from build123d import *

# Parameters (mm, degrees)
SKETCH_1_W                  = 56
SKETCH_1_H                  = 54
SKETCH_1_R                  = 5
EXTRUDE_1_DEPTH             = 9.2
HOLE_WIZARD_M2_1_AT_2_COUNT = 2
HOLE_WIZARD_M2_1_AT_2_PITCH = 48
HOLE_WIZARD_M2_1_AT_3_COUNT = 2
HOLE_WIZARD_M2_1_AT_3_PITCH = 46
HOLE_WIZARD_M2_1_AT_4_COUNT = 2
HOLE_WIZARD_M2_1_AT_4_PITCH = 66.483080554
SKETCH_13_W                 = 52.1
SKETCH_13_H                 = 50.1
CUT_EXTRUDE_1_DEPTH         = 40.558058597
SKETCH_14_W                 = 20
SKETCH_14_H                 = 13
CUT_EXTRUDE_2_DEPTH         = 40.970489114
SKETCH_15_R                 = 1.1
CUT_EXTRUDE_4_DEPTH         = 40.970489114
CUT_EXTRUDE_7_REACH         = 63.519
SKETCH_18_W                 = 5
SKETCH_18_H                 = 5
CUT_EXTRUDE_8_REACH         = 64.846
SKETCH_20_W                 = 17.8
SKETCH_20_H                 = 6
CUT_EXTRUDE_9_REACH         = 64.846
SKETCH_23_W                 = 20.32
SKETCH_23_H                 = 6
CHAMFER_1_SIZE              = 0.5
CUT_EXTRUDE_10_REACH        = 63.519
FILLET_4_R                  = 1.5
CHAMFER_2_SIZE              = 0.5
CHAMFER_3_SIZE              = 0.5
CUT_EXTRUDE_11_REACH        = 63.519
SKETCH_25_W                 = 5
SKETCH_25_H                 = 3.5
FILLET_5_R                  = 1.5
CUT_EXTRUDE_12_REACH        = 63.519
SKETCH_30_W                 = 6.5
SKETCH_30_H                 = 4.8
SKETCH_30_W_2               = 8
SKETCH_30_H_2               = 6
CUT_EXTRUDE_13_REACH        = 41.97
CHAMFER_4_SIZE              = 0.5
SKETCH_35_W                 = 7.974588705
SKETCH_35_H                 = 13
SKETCH_35_W_2               = 9
SKETCH_35_H_2               = 10.5
SKETCH_35_W_3               = 11
SKETCH_35_H_3               = 6.8
SKETCH_35_W_4               = 3.5
SKETCH_35_H_4               = 1.5
CUT_EXTRUDE_14_DEPTH        = 1.8
FILLET_6_R                  = 1.5


with BuildPart() as part:
    # 草图1 → 凸台-拉伸1 (new body)
    with BuildSketch(Plane(origin=(0, 0, 0), x_dir=(1, 0, 0), z_dir=(0, 1, 0))):
        Rectangle(SKETCH_1_W, SKETCH_1_H)
        with Locations(Location((0, 14, 0), (0, 0, 270))):
            Circle(SKETCH_1_R, mode=Mode.SUBTRACT)
    extrude(amount=EXTRUDE_1_DEPTH)

    # 草图6 → M2 六角圆柱头螺钉的柱形沉头孔1 (revolve, cut)
    with BuildSketch(Plane(origin=(-24, 9.2, -23), x_dir=(0, 0, 1), z_dir=(1, 0, 0))):
        Polygon((0, 0), (0, 9.2), (1.3, 9.2), (1.3, 2.3), (2.15, 2.3), (2.15, 0.025), (2.175, 0), align=None)
    hole_wizard_m2_1 = revolve(axis=Axis((-24, 15.55, -23), (0, -1, 0)), mode=Mode.SUBTRACT)

    # M2 六角圆柱头螺钉的柱形沉头孔1 at 2: M2 六角圆柱头螺钉的柱形沉头孔1 ×2
    with Locations(*[(i * HOLE_WIZARD_M2_1_AT_2_PITCH, 0, 0) for i in range(1, HOLE_WIZARD_M2_1_AT_2_COUNT)]):
        add(hole_wizard_m2_1, mode=Mode.SUBTRACT)

    # M2 六角圆柱头螺钉的柱形沉头孔1 at 3: M2 六角圆柱头螺钉的柱形沉头孔1 ×2
    with Locations(*[(0, 0, i * HOLE_WIZARD_M2_1_AT_3_PITCH) for i in range(1, HOLE_WIZARD_M2_1_AT_3_COUNT)]):
        add(hole_wizard_m2_1, mode=Mode.SUBTRACT)

    # M2 六角圆柱头螺钉的柱形沉头孔1 at 4: M2 六角圆柱头螺钉的柱形沉头孔1 ×2
    with Locations(*[Vector(0.7219882051154243, 0, 0.6919053632356149) * (i * HOLE_WIZARD_M2_1_AT_4_PITCH) for i in range(1, HOLE_WIZARD_M2_1_AT_4_COUNT)]):
        add(hole_wizard_m2_1, mode=Mode.SUBTRACT)

    # 草图13 → 切除-拉伸1 (cut, through all)
    with BuildSketch(Plane(origin=(0, 7.2, 0), x_dir=(1, 0, 0), z_dir=(0, 1, 0))):
        Rectangle(SKETCH_13_W, SKETCH_13_H)
    extrude(amount=-CUT_EXTRUDE_1_DEPTH, mode=Mode.SUBTRACT)

    # 草图14 → 切除-拉伸2 (cut, through all)
    with BuildSketch(Plane(origin=(0, 9.2, 0), x_dir=(1, 0, 0), z_dir=(0, 1, 0))):
        with Locations((2, -1.5)):
            Rectangle(SKETCH_14_W, SKETCH_14_H)
    extrude(amount=-CUT_EXTRUDE_2_DEPTH, mode=Mode.SUBTRACT)

    # 草图15 → 切除-拉伸4 (cut, through all)
    with BuildSketch(Plane(origin=(0, 9.2, 0), x_dir=(1, 0, 0), z_dir=(0, 1, 0))):
        with Locations(Location((16.5, 1.39, 0), (0, 0, 270))):
            Circle(SKETCH_15_R)
        with Locations(Location((16.5, -5.09, 0), (0, 0, 270))):
            Circle(SKETCH_15_R)
    extrude(amount=-CUT_EXTRUDE_4_DEPTH, mode=Mode.SUBTRACT)

    # 草图18 → 切除-拉伸7 (cut, up to next)
    with BuildSketch(Plane(origin=(0, 0, -27), x_dir=(-1, 0, 0), z_dir=(0, 0, -1)), mode=Mode.PRIVATE) as cut_extrude_7_sk1:
        with Locations((-3.5, 2.5)):
            Rectangle(SKETCH_18_W, SKETCH_18_H)
    cut_extrude_7_tool1 = extrude(cut_extrude_7_sk1.sketch, amount=-CUT_EXTRUDE_7_REACH, mode=Mode.PRIVATE) & part.part
    # 草图18 → 切除-拉伸7 (cut, up to next)
    with BuildSketch(Plane(origin=(0, 0, -27), x_dir=(-1, 0, 0), z_dir=(0, 0, -1)), mode=Mode.PRIVATE) as cut_extrude_7_sk2:
        with Locations((3.5, 2.5)):
            Rectangle(SKETCH_18_W, SKETCH_18_H)
    cut_extrude_7_tool2 = extrude(cut_extrude_7_sk2.sketch, amount=-CUT_EXTRUDE_7_REACH, mode=Mode.PRIVATE) & part.part
    add(cut_extrude_7_tool1.solids().sort_by_distance((3.5, 2.5, -27))[0], mode=Mode.SUBTRACT)
    add(cut_extrude_7_tool2.solids().sort_by_distance((-3.5, 2.5, -27))[0], mode=Mode.SUBTRACT)

    # 草图20 → 切除-拉伸8 (cut, up to next)
    with BuildSketch(Plane.ZY.offset(28), mode=Mode.PRIVATE) as cut_extrude_8_sk1:
        with Locations((-5.1, 3)):
            Rectangle(SKETCH_20_W, SKETCH_20_H)
    cut_extrude_8_tool1 = extrude(cut_extrude_8_sk1.sketch, amount=-CUT_EXTRUDE_8_REACH, mode=Mode.PRIVATE) & part.part
    add(cut_extrude_8_tool1.solids().sort_by_distance((-28, 3, -5.1))[0], mode=Mode.SUBTRACT)

    # 草图23 → 切除-拉伸9 (cut, up to next)
    with BuildSketch(Plane(origin=(28, 0, 0), x_dir=(0, 0, -1), z_dir=(1, 0, 0)), mode=Mode.PRIVATE) as cut_extrude_9_sk1:
        with Locations((6.33, 3)):
            Rectangle(SKETCH_23_W, SKETCH_23_H)
    cut_extrude_9_tool1 = extrude(cut_extrude_9_sk1.sketch, amount=-CUT_EXTRUDE_9_REACH, mode=Mode.PRIVATE) & part.part
    add(cut_extrude_9_tool1.solids().sort_by_distance((28, 3, -6.33))[0], mode=Mode.SUBTRACT)

    # 倒角1
    chamfer_1_edges = [part.edges().sort_by_distance(p)[0] for p in [
        (-8, 9.2, 1.5),
        (12, 9.2, 1.5),
    ]]
    chamfer(chamfer_1_edges, length=CHAMFER_1_SIZE)

    # 草图24 → 切除-拉伸10 (cut, up to next)
    with BuildSketch(Plane.XY.offset(27), mode=Mode.PRIVATE) as cut_extrude_10_sk1:
        with BuildLine():
            Line((-19.91, 6), (-14.17, 6))
            ThreePointArc((-14.17, 6), (-12.72, 4.55), (-14.17, 3.1))
            Line((-14.17, 3.1), (-19.91, 3.1))
            ThreePointArc((-19.91, 3.1), (-21.36, 4.55), (-19.91, 6))
        make_face()
    cut_extrude_10_tool1 = extrude(cut_extrude_10_sk1.sketch, amount=-CUT_EXTRUDE_10_REACH, mode=Mode.PRIVATE) & part.part
    add(cut_extrude_10_tool1.solids().sort_by_distance((-17.04, 4.55, 27))[0], mode=Mode.SUBTRACT)

    # 圆角4
    fillet_4_edges = [part.edges().sort_by_distance(p)[0] for p in [
        (1, 5, -26.025),
        (6, 5, -26.025),
        (-6, 5, -26.025),
        (-1, 5, -26.025),
    ]]
    fillet(fillet_4_edges, radius=FILLET_4_R)

    # 倒角2
    chamfer_2_edges = [part.edges().sort_by_distance(p)[0] for p in [
        (28, 3, 3.83),
        (28, 3, -16.49),
    ]]
    chamfer(chamfer_2_edges, length=CHAMFER_2_SIZE)

    # 倒角3
    chamfer_3_edges = [part.edges().sort_by_distance(p)[0] for p in [
        (-28, 3, 3.8),
        (-28, 3, -14),
    ]]
    chamfer(chamfer_3_edges, length=CHAMFER_3_SIZE)

    # 草图25 → 切除-拉伸11 (cut, up to next)
    with BuildSketch(Plane.XY.offset(27), mode=Mode.PRIVATE) as cut_extrude_11_sk1:
        with Locations((-10, 1.75)):
            Rectangle(SKETCH_25_W, SKETCH_25_H)
    cut_extrude_11_tool1 = extrude(cut_extrude_11_sk1.sketch, amount=-CUT_EXTRUDE_11_REACH, mode=Mode.PRIVATE) & part.part
    # 草图25 → 切除-拉伸11 (cut, up to next)
    with BuildSketch(Plane.XY.offset(27), mode=Mode.PRIVATE) as cut_extrude_11_sk2:
        with Locations((10, 1.75)):
            Rectangle(SKETCH_25_W, SKETCH_25_H)
    cut_extrude_11_tool2 = extrude(cut_extrude_11_sk2.sketch, amount=-CUT_EXTRUDE_11_REACH, mode=Mode.PRIVATE) & part.part
    # 草图25 → 切除-拉伸11 (cut, up to next)
    with BuildSketch(Plane.XY.offset(27), mode=Mode.PRIVATE) as cut_extrude_11_sk3:
        with Locations((0, 1.75)):
            Rectangle(SKETCH_25_W, SKETCH_25_H)
    cut_extrude_11_tool3 = extrude(cut_extrude_11_sk3.sketch, amount=-CUT_EXTRUDE_11_REACH, mode=Mode.PRIVATE) & part.part
    add(cut_extrude_11_tool1.solids().sort_by_distance((-10, 1.75, 27))[0], mode=Mode.SUBTRACT)
    add(cut_extrude_11_tool2.solids().sort_by_distance((10, 1.75, 27))[0], mode=Mode.SUBTRACT)
    add(cut_extrude_11_tool3.solids().sort_by_distance((0, 1.75, 27))[0], mode=Mode.SUBTRACT)

    # 圆角5
    fillet_5_edges = [part.edges().sort_by_distance(p)[0] for p in [
        (-12.5, 3.5, 26.025),
        (-7.5, 3.5, 26.025),
        (12.5, 3.5, 26.025),
        (7.5, 3.5, 26.025),
        (-2.5, 3.5, 26.025),
        (2.5, 3.5, 26.025),
    ]]
    fillet(fillet_5_edges, radius=FILLET_5_R)

    # 草图30 → 切除-拉伸12 (cut, up to next)
    with BuildSketch(Plane(origin=(0, 0, -27), x_dir=(-1, 0, 0), z_dir=(0, 0, -1)), mode=Mode.PRIVATE) as cut_extrude_12_sk1:
        with Locations((-14, 3.6)):
            Rectangle(SKETCH_30_W, SKETCH_30_H)
    cut_extrude_12_tool1 = extrude(cut_extrude_12_sk1.sketch, amount=-CUT_EXTRUDE_12_REACH, mode=Mode.PRIVATE) & part.part
    # 草图30 → 切除-拉伸12 (cut, up to next)
    with BuildSketch(Plane(origin=(0, 0, -27), x_dir=(-1, 0, 0), z_dir=(0, 0, -1)), mode=Mode.PRIVATE) as cut_extrude_12_sk2:
        with Locations((16.3, 3)):
            Rectangle(SKETCH_30_W_2, SKETCH_30_H_2)
    cut_extrude_12_tool2 = extrude(cut_extrude_12_sk2.sketch, amount=-CUT_EXTRUDE_12_REACH, mode=Mode.PRIVATE) & part.part
    add(cut_extrude_12_tool1.solids().sort_by_distance((14, 3.6, -27))[0], mode=Mode.SUBTRACT)
    add(cut_extrude_12_tool2.solids().sort_by_distance((-16.3, 3, -27))[0], mode=Mode.SUBTRACT)

    # 草图33 → 切除-拉伸13 (cut, up to next)
    with BuildSketch(Plane(origin=(0, 9.2, 0), x_dir=(1, 0, 0), z_dir=(0, 1, 0)), mode=Mode.PRIVATE) as cut_extrude_13_sk1:
        with BuildLine():
            Line((-2.85, 7.4), (-2.85, 6.3))
            ThreePointArc((-2.85, 6.3), (-3.6, 5.55), (-4.35, 6.3))
            Line((-4.35, 6.3), (-4.35, 7.4))
            ThreePointArc((-4.35, 7.4), (-3.6, 8.15), (-2.85, 7.4))
        make_face()
    cut_extrude_13_tool1 = extrude(cut_extrude_13_sk1.sketch, amount=-CUT_EXTRUDE_13_REACH, mode=Mode.PRIVATE) & part.part
    # 草图33 → 切除-拉伸13 (cut, up to next)
    with BuildSketch(Plane(origin=(0, 9.2, 0), x_dir=(1, 0, 0), z_dir=(0, 1, 0)), mode=Mode.PRIVATE) as cut_extrude_13_sk2:
        with BuildLine():
            Line((0.95, 7.4), (0.95, 6.3))
            ThreePointArc((0.95, 6.3), (0.2, 5.55), (-0.55, 6.3))
            Line((-0.55, 6.3), (-0.55, 7.4))
            ThreePointArc((-0.55, 7.4), (0.2, 8.15), (0.95, 7.4))
        make_face()
    cut_extrude_13_tool2 = extrude(cut_extrude_13_sk2.sketch, amount=-CUT_EXTRUDE_13_REACH, mode=Mode.PRIVATE) & part.part
    # 草图33 → 切除-拉伸13 (cut, up to next)
    with BuildSketch(Plane(origin=(0, 9.2, 0), x_dir=(1, 0, 0), z_dir=(0, 1, 0)), mode=Mode.PRIVATE) as cut_extrude_13_sk3:
        with BuildLine():
            Line((4.75, 7.4), (4.75, 6.3))
            ThreePointArc((4.75, 6.3), (4, 5.55), (3.25, 6.3))
            Line((3.25, 6.3), (3.25, 7.4))
            ThreePointArc((3.25, 7.4), (4, 8.15), (4.75, 7.4))
        make_face()
    cut_extrude_13_tool3 = extrude(cut_extrude_13_sk3.sketch, amount=-CUT_EXTRUDE_13_REACH, mode=Mode.PRIVATE) & part.part
    add(cut_extrude_13_tool1.solids().sort_by_distance((-3.6, 9.2, -6.85))[0], mode=Mode.SUBTRACT)
    add(cut_extrude_13_tool2.solids().sort_by_distance((0.2, 9.2, -6.85))[0], mode=Mode.SUBTRACT)
    add(cut_extrude_13_tool3.solids().sort_by_distance((4, 9.2, -6.85))[0], mode=Mode.SUBTRACT)

    # 倒角4
    chamfer_4_edges = [part.edges().sort_by_distance(p)[0] for p in [
        (-12.3, 3, -27),
        (-20.3, 3, -27),
    ]]
    chamfer(chamfer_4_edges, length=CHAMFER_4_SIZE)

    # 草图35 → 切除-拉伸14 (cut)
    with BuildSketch(Plane.XZ.offset(-7.2)):
        with Locations((16.631295972, 1.5)):
            Rectangle(SKETCH_35_W, SKETCH_35_H)
        with Locations((-5.5, 13.25)):
            Rectangle(SKETCH_35_W_2, SKETCH_35_H_2)
        with Locations((-16.7, 20.4)):
            Rectangle(SKETCH_35_W_3, SKETCH_35_H_3)
        with Locations((-16.3, -15.3)):
            Rectangle(SKETCH_35_W_4, SKETCH_35_H_4)
    extrude(amount=-CUT_EXTRUDE_14_DEPTH, mode=Mode.SUBTRACT)

    # 圆角6
    fillet_6_edges = [part.edges().sort_by_distance(p)[0] for p in [
        (28, 4.6, 27),
        (-28, 4.6, 27),
        (-28, 4.6, -27),
        (28, 4.6, -27),
    ]]
    fillet(fillet_6_edges, radius=FILLET_6_R)


solid = part.part
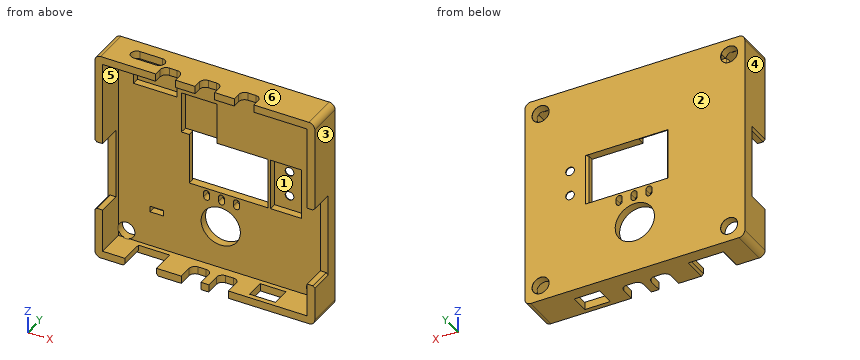
Build history of the part. All positions in model axes, mm. Face numbers are marked on the shaded views. A direction names the side the tool comes from. Round coordinates to 2 decimals unless told otherwise and drop trailing zeros. Write each loop counter-clockwise with the first axis right and the second up, starting at its lowest first coordinate (ties: lowest second). Pieces come first, ordered by that corner, then holes. Notation, with made-up numbers: (79, 41) - (132, 41) arc R10 cw to (132, 54) - close; hole circle Ø6 at (72.25, -26). An arc over 180 degrees is marked (long way). One line per question, with ' | ' between items.
1. Mould opens along X. For the marked faces 1, 2, 3 and 4 say: released by +X, released by -X, zero draft, split by the parting line, or undercut.
Results are:
face 1: undercut | face 2: zero draft | face 3: released by +X | face 4: released by -X
2. Band-saw the part on A-A, the plane x = 16.5. Write the cut outline in (y, z).
Results are:
outline: (0, -27) - (1.2, -27) - (1.2, -25.05) - (0, -25.05) - close; (0, 25.05) - (7.2, 25.05) - (7.2, 8) - (9, 8) - (9, 6.19) - (9.2, 6.19) - (9.2, 27) - (0, 27) - close; (6, -27) - (9.2, -27) - (9.2, -2.49) - (9, -2.49) - (9, -5) - (7.2, -5) - (7.2, -25.05) - (6, -25.05) - close; (9, -0.29) - (9.2, -0.29) - (9.2, 3.99) - (9, 3.99) - close
3. Drill centre lines: line 1 along X through (y, z) = (8.35, 23); line 2 along X through (y, z) = (1, 25.5); line 3 along X through (y, z) = (8.65, -23). Where is each one in solid material? Low to high. Write a range as from..to.
Results are:
line 1: -28..-26.15, -11.2..21.85, 26.15..28 | line 2: -28..-12.5, -7.5..-2.5, 2.5..7.5, 12.5..28 | line 3: -28..-26.15, -21.85..21.85, 26.15..28
4. Tool access for the marked faces 5 and 6: list every direction of +Z, -Z, +X, -X, +Y, -Y with a clear straight run to the whole face (end or side of a thin tool).
Results are:
face 5: -Y | face 6: +Z, +X, -X, +Y, -Y
5. Band-saw the part on B-B, the plane z = 23. Write the cut outline in (x, y) (3 decimals).
Results are:
outline: (-28, 0) - (-26.05, 0) - (-26.05, 6.9) - (-26.15, 6.9) - (-26.15, 9.175) - (-26.175, 9.2) - (-28, 9.2) - close; (-21.85, 9) - (-11.2, 9) - (-11.2, 7.2) - (21.85, 7.2) - (21.85, 9.175) - (21.825, 9.2) - (-21.825, 9.2) - (-21.85, 9.175) - close; (26.05, 0) - (28, 0) - (28, 9.2) - (26.175, 9.2) - (26.15, 9.175) - (26.15, 6.9) - (26.05, 6.9) - close
6. Band-saw the part on D-D, the plane z = 16. Write the cut outline in (x, y).
Results are:
outline: (-28, 0) - (-26.05, 0) - (-26.05, 7.2) - (-10, 7.2) - (-10, 9) - (-1, 9) - (-1, 7.2) - (26.05, 7.2) - (26.05, 0) - (28, 0) - (28, 9.2) - (-28, 9.2) - close
7. Band-saw the part on C-C, the plane x = 24. Write the cut outline in (y, z) (3 decimals), and give its area (3 significant figures).
Results are:
outline: (0, -27) - (9.2, -27) - (9.2, -25.175) - (9.175, -25.15) - (6.9, -25.15) - (6.9, -25.05) - (0, -25.05) - close; (0, 25.05) - (6.9, 25.05) - (6.9, 25.15) - (9.175, 25.15) - (9.2, 25.175) - (9.2, 27) - (0, 27) - close; (7.2, -20.85) - (9.175, -20.85) - (9.2, -20.825) - (9.2, 20.825) - (9.175, 20.85) - (7.2, 20.85) - close | area: 119 mm^2
8. Drop flat-ended pins along their axis: pin 1 Ø2 at (x, z) = (27.5, -4) entering from -Y; pin 2 Ø1 at (x, z) = (5, -15.5) entering from -Y; pin 3 Ø1.6 at (x, z) = (0.5, 25.5) entering from -Y. Give the stop position or say it passes through.
Results are:
pin 1: y = 6 | pin 2: y = 7.2 | pin 3: y = 3.47
